Input: dimensioned drawing with shaded views. Units: mm. Origin: part minimum x, y, z. A direction names the side the tool comes from. Round coordinates to 2 decimals unless told otherwise and drop trailing zeros. Write each loop counter-clockwise with the first axis right and the second up, starting at its lowest first coordinate (ties: lowest second). Pieces come first, ordered by that corner, then holes. Notation, with made-up numbers: M 65,13 L 101,13 A20 cw 101,51 Z; hole C 12,22.5 d2. An arc over 180 degrees is marked long. Answer in a Markdown table with one row per item. Add a question column.
Item 1: Cut plane A-A on y = 153. Return loops of the section in (x, z).
Item 2: Set-up query: the marked faces 1 and 2. Return all of +Z, -Z, +X, -X, +Y, -Y with unobstructed straight access to the full face (end or side cutting, diameter ignored); none if empty.
Item 3: Material intervals for probe 1 along X at (y, z) = (137.5, 732.5); probe 2 along Y at (x, z) = (192, 375.5), sorted ascending.
Item 4: Cut plane B-B on z = 786.5. Return loops of the section in (x, y), and give its area (3 significant figures).
Item 5: Mould query, pull axis X, two halves, no side actions, for the marked faces 3, 4 and 5. Classes: released by +X, released by -X, zero draft, split by the parting line, or undercut.
Item 6: Contact query for a flat-ended pin moving along its axis: pin 1 (8 mm diameter, centred on x = 76, z = 549, fed in from -Y). Output: stop coordinate, or through.
Item 7: Cut plane C-C on x = 281.5. Return loops of the section in (y, z).
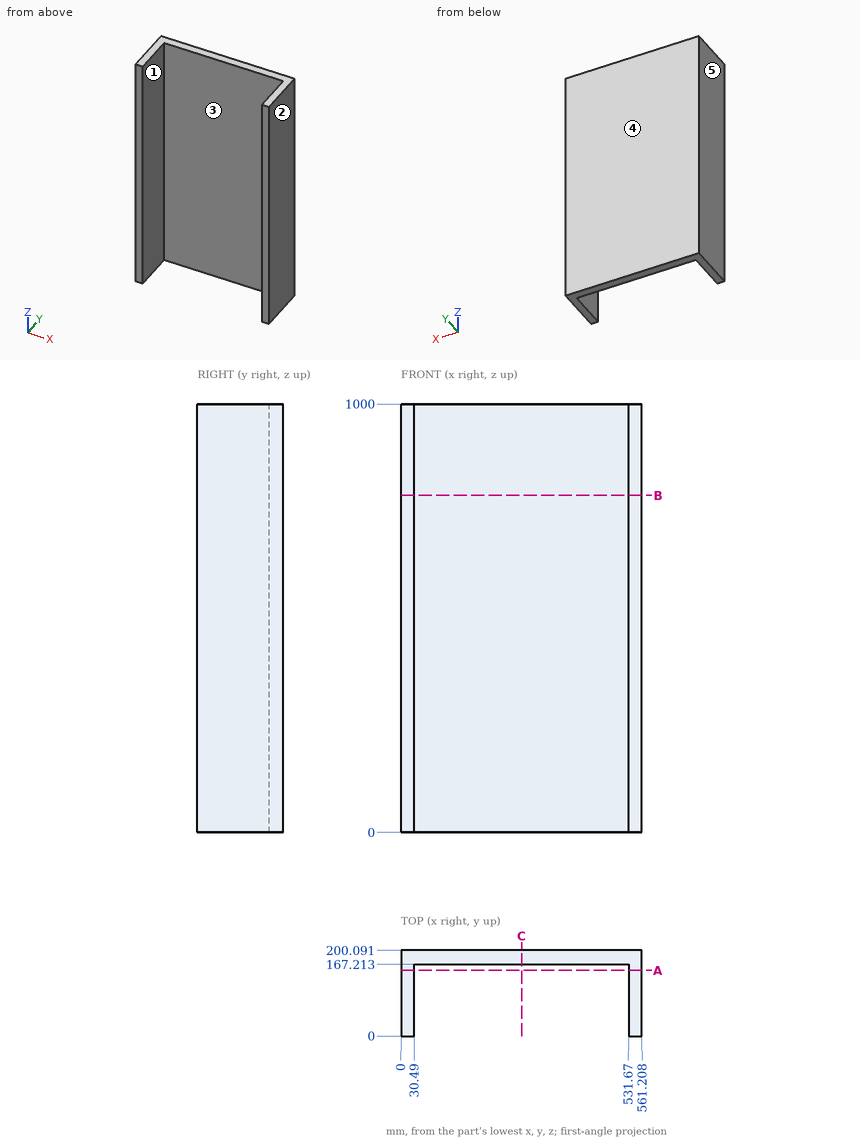
Results below:
| question | item | result |
|---|---|---|
| 1 | outline | M 0,0 L 30.49,0 L 30.49,1000 L 0,1000 Z; M 531.67,0 L 561.21,0 L 561.21,1000 L 531.67,1000 Z |
| 2 | face 1 | +Z, -Z, -Y |
| 2 | face 2 | +Z, -Z, +X, +Y, -Y |
| 3 | probe 1 | 0 to 30.49, 531.67 to 561.21 |
| 3 | probe 2 | 167.21 to 200.09 |
| 4 | outline | M 0,0 L 30.49,0 L 30.49,167.21 L 531.67,167.21 L 531.67,0 L 561.21,0 L 561.21,200.09 L 0,200.09 Z |
| 4 | area | 28,500 mm2 |
| 5 | face 3 | undercut |
| 5 | face 4 | zero draft |
| 5 | face 5 | released by -X |
| 6 | pin 1 | y = 167.21 |
| 7 | outline | M 167.21,0 L 200.09,0 L 200.09,1000 L 167.21,1000 Z |
